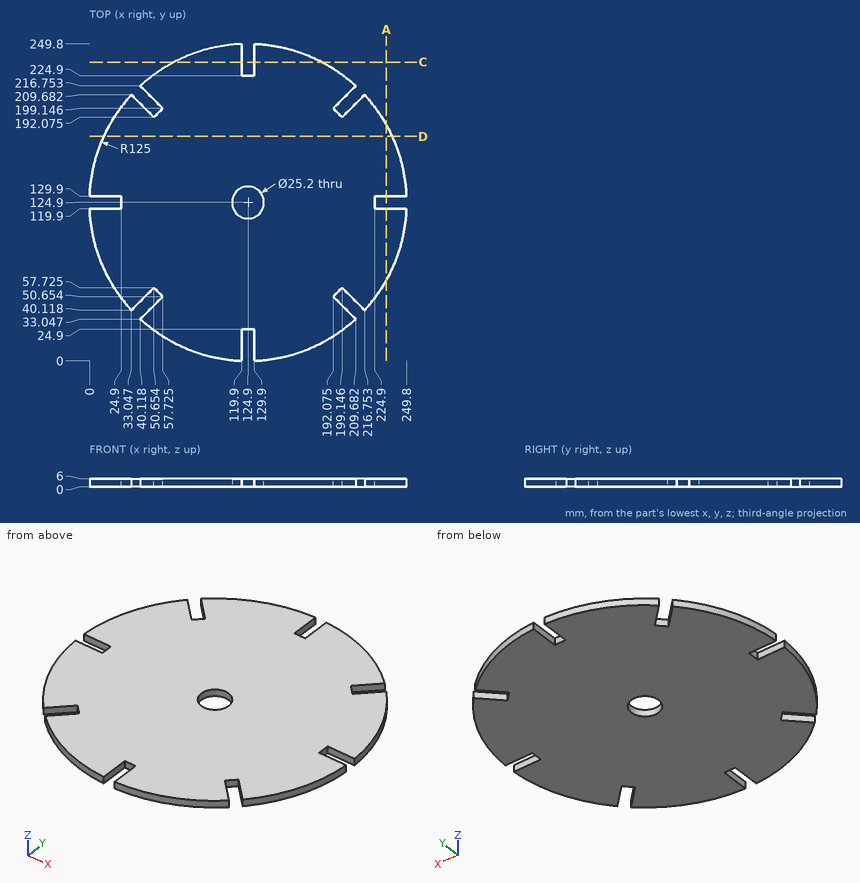
The drawing under review shows one solid part. Ordinate dimensions are in mm from its lowest x, y, z. Give positions to 0.01 mm unless a question says otherwise; leave off trailing zeros. Loops run counter-clockwise (first coordinate to the right, second up) from the corner with the lowest first, then second, coordinate; pieces in that order, holes last. Notation, with made-up numbers: M 79.25,48 L 91.25,48 A32 ccw 91.25,83 Z; hole C 71,62.25 d8. An arc over 180 degrees is marked long. Return JSON: item names as keys, results as strings. Group by question number.
Item 1: We need section A-A (x = 234). Give the boundary of the cut face in (y, z).
Item 2: Insertion check: pin 1 Ø1.8 at (x, z) = (124.5, 2) entering from -Y; pin 2 Ø10 at (x, y) = (129.5, 149) entering from -Z; pin 3 Ø1.8 at (y, z) = (127, 2) entering from -X; pin 4 Ø3 at (x, z) = (126.5, 3.5) entering from +Y. Each pin has a flat end and moves straight along its axis. Give the tip position at first contact, or say it passes through.
Item 3: We need section D-D (y = 177). Give the boundary of the cut face in (x, z) (1 decimal), and give its area (3 significant figures).
Item 4: For probe 1 along Y at (x, z) = (193, 1.6); probe 2 along Y at (x, z) = (49.5, 4); probe 3 along Y at (x, z) = (126, 3.25), list the stretches that pass through material, from the lowest coordinate up.
Item 5: We need section C-C (y = 235.5). Give the boundary of the cut face in (x, z).
Output:
{
 "1": {"outline": "M 63.89,0 L 119.9,0 L 119.9,6 L 63.89,6 Z; M 129.9,0 L 185.91,0 L 185.91,6 L 129.9,6 Z"},
 "2": {"pin 1": "stops at y = 24.9", "pin 2": "stops at z = 0", "pin 3": "stops at x = 24.9", "pin 4": "stops at y = 224.9"},
 "3": {"outline": "M 11.3,0 L 238.5,0 L 238.5,6 L 11.3,6 Z", "area": "1,360 mm^2"},
 "4": {"probe 1": "y = 20.08 to 49.73, 51.58 to 198.22, 200.07 to 229.72", "probe 2": "y = 25.2 to 42.43, 56.57 to 193.23, 207.37 to 224.6", "probe 3": "y = 24.9 to 112.35, 137.45 to 224.9"},
 "5": {"outline": "M 66.65,0 L 119.9,0 L 119.9,6 L 66.65,6 Z; M 129.9,0 L 183.15,0 L 183.15,6 L 129.9,6 Z"}
}
